```python
from build123d import *

# Parameters (mm, degrees)
F0_W     = 508
F0_H     = 381
F1_DEPTH = 76.2
F2_W     = 101.6
F2_H     = 254
F3_DEPTH = 76.2
F4_T     = -6.35
F5_W     = 114.3
F5_H     = 266.7
F6_DEPTH = 69.85


with BuildPart() as f1:
    # F0 (on Top) → F1 (new body)
    with BuildSketch(Plane.XY):
        Rectangle(F0_W, F0_H)
    extrude(amount=F1_DEPTH)

    # F2 (on face) → F3 (cut, through all)
    with BuildSketch(Plane.XY.offset(76.2)):
        with Locations((-152.4, 0)):
            Rectangle(F2_W, F2_H)
    extrude(amount=-F3_DEPTH, mode=Mode.SUBTRACT)

    # F4
    f4_openings = [f1.faces().sort_by_distance(p)[0] for p in [
        (23.446154, 0, 76.2),
    ]]
    offset(amount=F4_T, openings=f4_openings)

    # F5 (on face) → F6 (cut)
    with BuildSketch(Plane.XY.offset(76.2)):
        with Locations((-152.4, 0)):
            Rectangle(F5_W, F5_H)
    extrude(amount=-F6_DEPTH, mode=Mode.SUBTRACT)


solid = f1.part
```
Model file for the job. Use its own axes, mm. A direction names the side the tool comes from. Give positions to 0.01 mm unless a question says otherwise; leave off trailing zeros. Write each loop counter-clockwise with the first axis right and the second up, starting at its lowest first coordinate (ties: lowest second). Pieces come first, ordered by that corner, then holes. Notation, with made-up numbers: (-35.5, 3.5) - (-4.5, 3.5) arc R24 cw to (-4.5, 15.5) - close; hole circle Ø3 at (70, 19.5). An arc over 180 degrees is marked (long way). One line per question, with ' | ' between items. Start each with the question number.
(1) 3-axis set-ups, long thin cutter, end or side, ignore diameter. For faces 1 (the face through (-247.65, -3, 41)), 2 (the face through (-4, -190.5, 38)): which of +Z, -Z, +X, -X, +Y, -Y reach the whole face in a straight line?
(2) Slice it at D-D on y = -159.5. Write the cut outline in (x, z).
(3) Slice it at C-C on z = 16. Write the cut outline in (x, y), plus the area to 3 significant figures.
(4) Two-plate mould, pull along X, no slides. Class faces 3 (the face through (52, 3, 6.35)), 4 (the face through (-4, 3, 0)), 5 (the face through (-254, -3, 38)), 6 (the face through (254, -3, 38)): +X half, -X half, draft (parallel to the pull), parting line (faces both ways), or undercut.
(5) Slice it at A-A on y = -23.5. Write the cut outline in (x, z).
(6) Slice it at B-B on x = -176.5. Write the cut outline in (y, z), plus the area to 3 significant figures.
(7) Wall check: line 1 along X through (y, z) = (-129.5, 9); line 2 along Y through (x, z) = (-175, 8.5). Give the ranges that are in metal, low to high. Write a range as from..to.
Results below:
1) face 1: +Z | face 2: +Z, -Z, +X, -X, -Y
2) outline: (-254, 0) - (254, 0) - (254, 76.2) - (247.65, 76.2) - (247.65, 6.35) - (-247.65, 6.35) - (-247.65, 76.2) - (-254, 76.2) - close
3) outline: (-254, -190.5) - (254, -190.5) - (254, 190.5) - (-254, 190.5) - close; hole (-247.65, -184.15) - (247.65, -184.15) - (247.65, 184.15) - (-247.65, 184.15) - close | area: 11,100 mm^2
4) face 3: undercut | face 4: draft | face 5: -X half | face 6: +X half
5) outline: (-254, 0) - (-203.2, 0) - (-203.2, 6.35) - (-247.65, 6.35) - (-247.65, 76.2) - (-254, 76.2) - close; (-101.6, 0) - (254, 0) - (254, 76.2) - (247.65, 76.2) - (247.65, 6.35) - (-101.6, 6.35) - close
6) outline: (-190.5, 0) - (-127, 0) - (-127, 6.35) - (-184.15, 6.35) - (-184.15, 76.2) - (-190.5, 76.2) - close; (127, 0) - (190.5, 0) - (190.5, 76.2) - (184.15, 76.2) - (184.15, 6.35) - (127, 6.35) - close | area: 1,690 mm^2
7) line 1: -254..-247.65, 247.65..254 | line 2: -190.5..-184.15, 184.15..190.5
